Geometry: final body of the model. Coordinates: model frame, mm. A direction names the side the tool comes from. Coordinates: 2 decimals unless noted, no trailing zeros. Write each loop counter-clockwise with the first axis right and the second up, starting at its lowest first coordinate (ties: lowest second). Pieces come first, ordered by that corner, then holes. Notation, with made-up numbers: M 85.5,86 L 101.5,86 A18 ccw 101.5,93 Z; hole C 18.5,74.25 d2. An arc over 180 degrees is marked long. Write item = value, one per line. Start each with the question number.
Item 1: Ray query, L1, parallel to Y at x = 45.5, z = 60.5; L2, parallel to Z at x = 1.5, y = 135. Return the intervals inside material, ascending. Write a range as [from, to].
Item 2: First-contact query: pin 1 Ø8 at (x, z) = (8.5, 104.5) entering from +Y; pin 2 Ø4 at (x, y) = (3, 24.5) entering from +Z. Flat tips, straight axial feed; report the tip coordinate or a pass-through.
Item 3: Section B-B on y = 78.5. Output: boundary loops of the cut face in (x, z), plus the area to 3 significant figures.
Item 4: Pull-direction query (Y, two-part tool) for faces 1 (the flat face through (16, 18.589, 77)), 2 (the flat face through (16, -18.737, 64)), 3 (the flat face through (-21.036, 29, 20)); classes: +Y half, -Y half, draft (parallel to the pull), parting line (faces both ways), or undercut.
Item 5: Section A-A on x = 10. Output: boundary loops of the cut face in (y, z).
Item 6: Section C-C on z = 63. Output: boundary loops of the cut face in (x, y).
Item 7: Reachability of faces 4 (the flat face through (16, 0, 126.383)), 5 (the flat face through (16, 88, 25.4)) from +Z, -Z, +X, -X, +Y, -Y: full face, straight path, thin tool, end or side. Return the list, or none.
from build123d import *

# Parameters (mm, degrees)
F0_W     = 75.4162408412
F0_H     = 175.0652268529
F1_DEPTH = 25.4
F2_W     = 75.4162408412
F2_H     = 100.9825893402
F3_DEPTH = 37.3262315989


with BuildPart() as f1:
    # F0 (on Top) → F1 (new body)
    with BuildSketch(Plane.XY):
        with Locations((16.6725758463, 68.7957666814)):
            Rectangle(F0_W, F0_H)
    extrude(amount=F1_DEPTH)

    # F2 (on face) → F3 (join)
    with BuildSketch(Plane.XZ.offset(18.736846745)):
        with Locations((16.6725758463, 75.8912946701)):
            Rectangle(F2_W, F2_H)
    extrude(amount=-F3_DEPTH)


solid = f1.part
Responses:
q1.L1 = [-18.74, 18.59]
q1.L2 = [0, 25.4]
q2.pin_1 = 18.59
q2.pin_2 = 25.4
q3.outline = M -21.04,0 L 54.38,0 L 54.38,25.4 L -21.04,25.4 Z
q3.area = 1,920 mm²
q4.face_1 = +Y half
q4.face_2 = -Y half
q4.face_3 = draft
q5.outline = M -18.74,0 L 156.33,0 L 156.33,25.4 L 18.59,25.4 L 18.59,126.38 L -18.74,126.38 Z
q6.outline = M -21.04,-18.74 L 54.38,-18.74 L 54.38,18.59 L -21.04,18.59 Z
q7.face_4 = +Z, +X, -X, +Y, -Y
q7.face_5 = +Z, +X, -X, +Y
